Work out the finished part from the listing and answer in its coordinate system (mm). Coordinates: 2 decimals unless noted, no trailing zeros. Order: outer loops, then holes, each group sorted by start corner. A loop starts at its lowest first (then second) coordinate and runs counter-clockwise, first axis right, second up. Notation, with made-up numbers: M 77,19.5 L 122,19.5 A20 ccw 122,49.5 Z; hole C 81.5,2 d11. An arc over 180 degrees is marked long. Answer in a Markdown table with one row per item. Add a question column.
Item 1: The part is cut by section D-D (x = -25). Write down the section's boundary in (y, z), then the cut area to 3 significant figures.
Item 2: The part is cut by section C-C (y = 42.5). Write down the section's boundary in (x, z), then the cut area to 3 significant figures.
Item 3: Consider line 1 (Y direction, x = -33, z = 0.9); line 2 (X direction, y = -14.5, z = 3.4); line 3 (X direction, y = -17.5, z = 5.55). Determine where each line is inside the solid, lowest interval first. Write a range as from..to.
Item 4: The part is cut by section A-A (y = 0). Write down the section's boundary in (x, z).
Item 5: The part is cut by section B-B (z = 1.75). Write down the section's boundary in (x, y) (3 decimals), then the cut area to 3 significant figures.
Item 6: Flat-ended cylindrical pins translate along their axes: pin 1 Ø2.5 at (y, z) = (-21, 4) entering from -X; pin 2 Ø1.4 at (x, z) = (-31.5, 3) entering from -Y; pin 3 Ø0.9 at (y, z) = (-20.5, 4) entering from +X. Find the tip coordinate at first contact, or state that the pin passes through.
from build123d import *

# Parameters (mm, degrees)
CROQUIS1_R              = 49
SALIENTE_EXTRUIR1_DEPTH = 6
CROQUIS2_R              = 3
CORTAR_EXTRUIR1_DEPTH   = 10


with BuildPart() as part:
    # Croquis1 → Saliente-Extruir1 (new body)
    # profile 1 of 2: a face of its own
    with BuildSketch(Plane.XY):
        Circle(CROQUIS1_R)
        Polygon((-5, 36.339745962), (0, 45), (5, 36.339745962), (33.97114317, -13.839745962), (38.97114317, -22.5), (28.97114317, -22.5), (-28.97114317, -22.5), (-38.97114317, -22.5), (-33.97114317, -13.839745962), align=None, mode=Mode.SUBTRACT)
    # profile 2 of 2: a face of its own
    with BuildSketch(Plane.XY):
        Polygon((-2.401923789, 34.839745962), (-5, 36.339745962), (-33.97114317, -13.839745962), (-31.373066959, -15.339745962), (-33.774990748, -19.5), (-28.97114317, -19.5), (-28.97114317, -22.5), (28.97114317, -22.5), (28.97114317, -19.5), (33.774990748, -19.5), (31.373066959, -15.339745962), (33.97114317, -13.839745962), (5, 36.339745962), (2.401923789, 34.839745962), (0, 39), align=None)
    extrude(amount=SALIENTE_EXTRUIR1_DEPTH)

    # Croquis2 → Cortar-Extruir1 (cut)
    with BuildSketch(Plane.XY.offset(6)):
        with BuildLine():
            Line((-9.539392014, 3), (-14, 3))
            Line((-14, 3), (-14, -3))
            Line((-14, -3), (-9.539392014, -3))
            ThreePointArc((-9.539392014, -3), (-10, 0), (-9.539392014, 3))
        make_face()
        with BuildLine():
            Line((-6, 3), (-9.539392014, 3))
            ThreePointArc((-9.539392014, 3), (-10, 0), (-9.539392014, -3))
            Line((-9.539392014, -3), (-6, -3))
            Line((-6, -3), (-6, 3))
        make_face()
        Circle(CROQUIS2_R)
    extrude(amount=-CORTAR_EXTRUIR1_DEPTH, mode=Mode.SUBTRACT)


solid = part.part
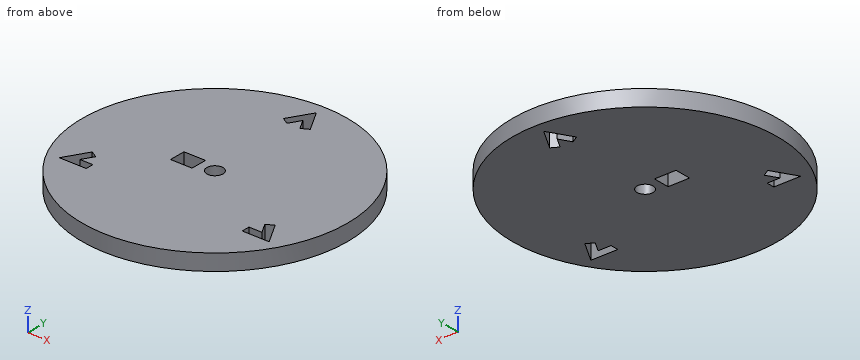
Reply:
| question | item | result |
|---|---|---|
| 1 | outline | M -42.14,0 L 42.14,0 L 42.14,6 L -42.14,6 Z |
| 1 | area | 506 mm2 |
| 2 | outline | M -24.39,0 L -1.44,0 L -1.44,6 L -24.39,6 Z; M 1.44,0 L 24.39,0 L 24.39,6 L 1.44,6 Z |
| 2 | area | 275 mm2 |
| 3 | line 1 | y = -36.22..-22.5, -19.5..-18.16, -14.4..36.22 |
| 3 | line 2 | x = -46.81..-34.35, -32.83..32.83, 34.35..46.81 |
| 3 | line 3 | x = -45.77..-36.08, -32.62..32.62, 36.08..45.77 |
| 4 | outline | M -49,0 L -14,0 L -14,6 L -49,6 Z; M -6,0 L -3,0 L -3,6 L -6,6 Z; M 3,0 L 49,0 L 49,6 L 3,6 Z |
| 5 | outline | C 0,0 d98; hole M -38.971,-22.5 L -28.971,-22.5 L -28.971,-19.5 L -33.775,-19.5 L -31.373,-15.34 L -33.971,-13.84 Z; hole M -14,-3 L -6,-3 L -6,3 L -14,3 Z; hole M -5,36.34 L -2.402,34.84 L 0,39 L 2.402,34.84 L 5,36.34 L 0,45 Z; hole C 0,0 d6; hole M 28.971,-22.5 L 38.971,-22.5 L 33.971,-13.84 L 31.373,-15.34 L 33.775,-19.5 L 28.971,-19.5 Z |
| 5 | area | 7,330 mm2 |
| 6 | pin 1 | stops at x = -44.84 |
| 6 | pin 2 | stops at y = -38.11 |
| 6 | pin 3 | stops at x = 44.71 |
